Can you work these out from the model? Positions are in its coordinate system, mm. A direction names the side the tool comes from. Give positions to 0.01 mm unless a question says otherwise; leave off trailing zeros. Order: outer loops, then holes, each group sorted by start corner. A loop starts at its lowest first (then second) coordinate and runs counter-clockwise, first axis right, second up. Notation, with made-up numbers: M -39,-37.5 L -32,-37.5 A20 cw -32,-16.5 Z; hole C 72.5,-10.5 d5. An arc over 180 degrees is marked long. Answer as a JSON object with one key per item and string values.
```python
from build123d import *

# Parameters (mm, degrees)
F1_DEPTH = 8
F2_R     = 6.35
F3_DEPTH = 8.001
F4_D     = 11.50874


with BuildPart() as f1:
    # F0 (on Top) → F1 (new body)
    with BuildSketch(Plane.XY):
        with BuildLine():
            Line((31.3706356287, 124.5844857395), (-93.6293643713, 124.5844857395))
            ThreePointArc((-93.6293643713, 124.5844857395), (-107.771499995, 118.7266213632), (-113.6293643713, 104.5844857395))
            Line((-113.6293643713, 104.5844857395), (-113.6293643713, -20.4155142605))
            ThreePointArc((-113.6293643713, -20.4155142605), (-107.771499995, -34.5576498843), (-93.6293643713, -40.4155142605))
            Line((-93.6293643713, -40.4155142605), (31.3706356287, -40.4155142605))
            ThreePointArc((31.3706356287, -40.4155142605), (45.5127712524, -34.5576498843), (51.3706356287, -20.4155142605))
            Line((51.3706356287, -20.4155142605), (51.3706356287, 104.5844857395))
            ThreePointArc((51.3706356287, 104.5844857395), (45.5127712524, 118.7266213632), (31.3706356287, 124.5844857395))
        make_face()
        with BuildLine():
            ThreePointArc((-83.6293643713, 79.5844857395), (-79.2359660891, 90.1910874573), (-68.6293643713, 94.5844857395))
            Line((-68.6293643713, 94.5844857395), (6.3706356287, 94.5844857395))
            ThreePointArc((6.3706356287, 94.5844857395), (16.9772373465, 90.1910874573), (21.3706356287, 79.5844857395))
            Line((21.3706356287, 79.5844857395), (21.3706356287, 4.5844857395))
            ThreePointArc((21.3706356287, 4.5844857395), (16.9772373465, -6.0221159783), (6.3706356287, -10.4155142605))
            Line((6.3706356287, -10.4155142605), (-68.6293643713, -10.4155142605))
            ThreePointArc((-68.6293643713, -10.4155142605), (-79.2359660891, -6.0221159783), (-83.6293643713, 4.5844857395))
            Line((-83.6293643713, 4.5844857395), (-83.6293643713, 79.5844857395))
        make_face(mode=Mode.SUBTRACT)
    extrude(amount=F1_DEPTH)

    # F2 (on face) → F3 (cut, through all)
    with BuildSketch(Plane.XY.offset(8)):
        with Locations((-93.6293643713, 104.5844857395)):
            Circle(F2_R)
        with Locations((-31.1293643713, 109.5844857395)):
            Circle(F2_R)
        with Locations((31.3706356287, 104.5844857395)):
            Circle(F2_R)
        with Locations((36.3706356287, 42.0844857395)):
            Circle(F2_R)
        with Locations((31.3706356287, -20.4155142605)):
            Circle(F2_R)
        with Locations((-31.1293643713, -25.4155142605)):
            Circle(F2_R)
        with Locations((-93.6293643713, -20.4155142605)):
            Circle(F2_R)
        with Locations((-98.6293643713, 42.0844857395)):
            Circle(F2_R)
    extrude(amount=-F3_DEPTH, mode=Mode.SUBTRACT)

    # F4 (through all)
    with Locations(Plane.XY.offset(8)):
        with Locations((-98.6293643713, 11.3532003015)):
            Hole(F4_D / 2)


solid = f1.part
```
1) I want a section at D-D on z = 2.5. Count the separate pieces of the cut face and the enclosed holes in it, and give its area (3 significant figures).
Results found:
{"separate pieces": "1", "enclosed holes": "10", "area": "14,900 mm²"}
2) I need wall thicknesses on L1, parallel to X at y = 12, z = 4.25; L2, parallel to Y at x = -3.5, z = 3.25; L3, parallel to X at y = 50, z = 3. Which ranges of each line are inside material? Lowest first, please.
Results found:
{"L1": "x = -113.63 to -104.35, -92.91 to -83.63, 21.37 to 51.37", "L2": "y = -40.42 to -10.42, 94.58 to 124.58", "L3": "x = -113.63 to -83.63, 21.37 to 51.37"}
3) I want a section at C-C on x = -102.5. Write out the boundary of the cut face in (y, z).
Results found:
{"outline": "M -38.34,0 L 7.1,0 L 7.1,8 L -38.34,8 Z; M 15.61,0 L 37.05,0 L 37.05,8 L 15.61,8 Z; M 47.12,0 L 122.51,0 L 122.51,8 L 47.12,8 Z"}
4) I want a section at A-A on x = -18. Write out the boundary of the cut face in (y, z), and give its area (3 significant figures).
Results found:
{"outline": "M -40.42,0 L -10.42,0 L -10.42,8 L -40.42,8 Z; M 94.58,0 L 124.58,0 L 124.58,8 L 94.58,8 Z", "area": "480 mm²"}
5) I want a section at B-B on y = 68. Write out the boundary of the cut face in (x, z).
Results found:
{"outline": "M -113.63,0 L -83.63,0 L -83.63,8 L -113.63,8 Z; M 21.37,0 L 51.37,0 L 51.37,8 L 21.37,8 Z"}
6) For faces 5 (the face through (-32, 98, 0)), 6 (the face through (17, -6, 4)), which set-ups out of +Z, -Z, +X, -X, +Y, -Y let a thin tool reach every point of the face, with its end or its side?
Results found:
{"face 5": "-Z, +X, -X, +Y, -Y", "face 6": "+Z, -Z"}
7) Thinking about a two-plate mould opening in X: for faces 1 (the face through (-32, 94.584, 4)), 2 (the face through (51.371, 41, 4)), 3 (the face through (-30, 124.584, 4)), 4 (the face through (-94.46, 110.88, 4.06)), which applies, pulls with the +X half, pulls with the -X half, needs draft (parallel to the pull), parting line crosses it, or undercut?
Results found:
{"face 1": "undercut", "face 2": "pulls with the +X half", "face 3": "needs draft", "face 4": "undercut"}
